Input: part model. Units: mm. Frame: model coordinates. A direction names the side the tool comes from. Give positions to 0.01 mm unless a question says otherwise; leave off trailing zeros.
from build123d import *

# Parameters (mm, degrees)
J1_COLLET_OUTER_PROFILE_W    = 17.8
J1_COLLET_OUTER_PROFILE_H    = 2
J1_COLLET_HEX_BORE_DEPTH     = 29.804166365
J1_COLLET_MASTER_SLIT_DEPTH  = 12
J1_COLLET_SLIT_PATTERN_COUNT = 6


with BuildPart() as part:
    # J1_Collet_Outer_Profile → J1_Collet_Blank (revolve)
    with BuildSketch(Plane.XY, mode=Mode.PRIVATE) as j1_collet_blank_sk:
        Polygon((16.113509984, 12), (0, 12), (0, 0), (17.8, 0), align=None)
        with Locations((8.9, -1)):
            Rectangle(J1_COLLET_OUTER_PROFILE_W, J1_COLLET_OUTER_PROFILE_H)
    revolve(j1_collet_blank_sk.sketch.rotate(Axis((0, 12, 0), (0, -1, 0)), 180), axis=Axis((0, 12, 0), (0, -1, 0)))

    # J1_Collet_Hex_Bore_Profile → J1_Collet_Hex_Bore (cut, through all)
    with BuildSketch(Plane.XZ.offset(2)):
        Polygon((15.386384674, 0), (7.693192337, 13.325), (-7.693192337, 13.325), (-15.386384674, 0), (-7.693192337, -13.325), (7.693192337, -13.325), align=None)
    extrude(amount=-J1_COLLET_HEX_BORE_DEPTH, mode=Mode.SUBTRACT)

    # J1_Collet_Master_Slit_Profile → J1_Collet_Master_Slit (cut)
    with BuildSketch(Plane(origin=(0, 12, 0), x_dir=(1, 0, 0), z_dir=(0, 1, 0))):
        Polygon((11.166583425, 6.908910162), (15.106160781, 9.183426209), (15.506160781, 8.490605886), (11.566583425, 6.216089838), align=None)
    j1_collet_master_slit = extrude(amount=-J1_COLLET_MASTER_SLIT_DEPTH, mode=Mode.SUBTRACT)

    # J1_Collet_Slit_Pattern: J1_Collet_Master_Slit ×6 about axis
    j1_collet_slit_pattern_axis = Axis((0, 0, 0), (0, 1, 0))
    for i in range(1, J1_COLLET_SLIT_PATTERN_COUNT):
        add(j1_collet_master_slit.rotate(j1_collet_slit_pattern_axis, i * 360 / J1_COLLET_SLIT_PATTERN_COUNT), mode=Mode.SUBTRACT)


solid = part.part
(1) Reachability of faces 1 (the flat face through (12.83, 6.08, 7.87)), 2 (the flat face through (15.9, 12, -0.1)), 3 (the flat face through (12.34, 4.9, -5.28)) from +Z, -Z, +X, -X, +Y, -Y: full face, straight path, thin tool, end or side. Return the list, or none.
Values follow:
face 1: +Y
face 2: +Z, -Z, +X, -X, +Y
face 3: +Y, -Y
(2) Cut plane A-A (y = 4.5). Count the separate pieces of the cut face and the enclosed holes in it, and give its area (3 significant figures).
Values follow:
separate pieces: 6
enclosed holes: 0
area: 292 mm2
(3) Ray query, probe 1 along X at (y, z) = (2.5, -8); probe 2 along X at (y, z) = (0.5, 4); probe 3 along Z at (x, y) = (2.5, 3.5) (3 decimals). Return the intervals inside material, ascending.
Values follow:
probe 1: x = -15.51 to -14.66, -13.06 to -10.77, 10.77 to 13.06, 14.66 to 15.51
probe 2: x = -17.27 to -13.08, 13.08 to 17.27
probe 3: z = -17.127 to -13.325, 13.325 to 17.127
(4) Mould query, pull axis Z, two halves, no side actions, for faces 4 (the cylindrical face through (13.12, -0.99, -12.03)), 5 (the flat face through (-12, -2, -7)), 6 (the flat face through (-13.4, 0, 7.8)), 7 (the flat face through (13.4, 0, 7.8)). Classes: +Z half, -Z half, draft (parallel to the pull), parting line (faces both ways), or undercut.
Values follow:
face 4: parting line
face 5: draft
face 6: undercut
face 7: undercut
(5) Pin query (flat end, axial travel): pin 1 Ø2 at (y, z) = (9, -16) entering from -X; pin 2 Ø4 at (x, y) = (6.5, 9) entering from +Z; pin 3 Ø5 at (y, z) = (3, 16) entering from -X. Return the tip coordinate at first contact, or that it passes through.
Values follow:
pin 1: stops at x = -6.98
pin 2: stops at z = 15.98
pin 3: stops at x = -10.99
